For this review, take the finished solid that the model builds, in its own axes (mm). A direction names the side the tool comes from. Coordinates: 2 decimals unless noted, no trailing zeros. Loops run counter-clockwise (first coordinate to the right, second up) from the corner with the lowest first, then second, coordinate; pieces in that order, holes last. Notation, with made-up numbers: (26.25, -19) -> (74.25, -19) arc R11 ccw to (74.25, -3) -> close; hole circle Ø4 at (47, 80.25). An arc over 180 degrees is marked (long way). Use a Markdown table: item, result.
from build123d import *

# Parameters (mm, degrees)
BOSS_EXTRUDE1_DEPTH = 8


with BuildPart() as part:
    # Sketch1 → Boss-Extrude1 (new body)
    with BuildSketch(Plane(origin=(0, 0, 0), x_dir=(1, 0, 0), z_dir=(0, 1, 0))):
        with BuildLine():
            Line((-6, 6), (6, 6))
            ThreePointArc((6, 6), (12, 0), (6, -6))
            Line((6, -6), (-6, -6))
            ThreePointArc((-6, -6), (-12, 0), (-6, 6))
        make_face()
        Polygon((-4.63382, 3.298250285), (-7.36618, 3.298250285), (-9.298250285, 1.36618), (-9.298250285, -1.36618), (-7.36618, -3.298250285), (-4.63382, -3.298250285), (-2.701749715, -1.36618), (-2.701749715, 1.36618), align=None, mode=Mode.SUBTRACT)
        Polygon((8.355898234, 0.975845), (6.975845, 2.355898234), (5.024155, 2.355898234), (3.644101766, 0.975845), (3.644101766, -0.975845), (5.024155, -2.355898234), (6.975845, -2.355898234), (8.355898234, -0.975845), align=None, mode=Mode.SUBTRACT)
    extrude(amount=BOSS_EXTRUDE1_DEPTH)


solid = part.part
(1) For pin 1 Ø1.5 at (x, z) = (-6.5, -3.5) entering from -Y; pin 2 Ø4 at (x, y) = (9.5, 4.5) entering from +Z; pin 3 Ø1 at (x, z) = (-7, 2) entering from -Y; pin 4 Ø0.6 at (y, z) = (3.5, -0.5) entering from +X, all flat-tipped, find the tip position at first contact; note any pin that passes through.
Found:
| item | result |
|---|---|
| pin 1 | stops at y = 0 |
| pin 2 | stops at z = 5.81 |
| pin 3 | passes through |
| pin 4 | stops at x = 12 |
(2) Take a section at D-D on z = 2.75. Write out the cut boundary in (x, y).
Found:
| item | result |
|---|---|
| outline | (-11.33, 0) -> (-7.91, 0) -> (-7.91, 8) -> (-11.33, 8) -> close; (-4.09, 0) -> (11.33, 0) -> (11.33, 8) -> (-4.09, 8) -> close |
(3) For line 1 along X through (y, z) = (7, -0.25); line 2 along Z through (x, y) = (6.25, 5.75); line 3 along X through (y, z) = (7, 1.75), list the stretches that pass through material, from the lowest coordinate up.
Found:
| item | result |
|---|---|
| line 1 | x = -11.99 to -9.3, -2.7 to 3.64, 8.36 to 11.99 |
| line 2 | z = -5.99 to -2.36, 2.36 to 5.99 |
| line 3 | x = -11.74 to -8.91, -3.09 to 4.42, 7.58 to 11.74 |
(4) Take a section at A-A on z = 0. Write out the cut boundary in (x, y), plus the area to 3 significant figures.
Found:
| item | result |
|---|---|
| outline | (-12, 0) -> (-9.3, 0) -> (-9.3, 8) -> (-12, 8) -> close; (-2.7, 0) -> (3.64, 0) -> (3.64, 8) -> (-2.7, 8) -> close; (8.36, 0) -> (12, 0) -> (12, 8) -> (8.36, 8) -> close |
| area | 102 mm^2 |
(5) For faces 1 (the face through (3.644, 4, 0)), 2 (the face through (12, 4, 0)), list the 3-axis set-ups (+Z, -Z, +X, -X, +Y, -Y) from which the entire face can be reached by the end or side of a thin tool; tool diameter is ignored.
Found:
| item | result |
|---|---|
| face 1 | +Y, -Y |
| face 2 | +X, +Y, -Y |
(6) Take a section at C-C on x = -8.25. Write out the cut boundary in (y, z), plus the area to 3 significant figures.
Found:
| item | result |
|---|---|
| outline | (0, -5.56) -> (8, -5.56) -> (8, -2.41) -> (0, -2.41) -> close; (0, 2.41) -> (8, 2.41) -> (8, 5.56) -> (0, 5.56) -> close |
| area | 50.4 mm^2 |
(7) Take a section at B-B on y = 2. Write out the cut boundary in (x, z).
Found:
| item | result |
|---|---|
| outline | (-6, -6) -> (6, -6) arc R6 ccw to (6, 6) -> (-6, 6) arc R6 ccw to start; hole (-9.3, -1.37) -> (-7.37, -3.3) -> (-4.63, -3.3) -> (-2.7, -1.37) -> (-2.7, 1.37) -> (-4.63, 3.3) -> (-7.37, 3.3) -> (-9.3, 1.37) -> close; hole (3.64, -0.98) -> (5.02, -2.36) -> (6.98, -2.36) -> (8.36, -0.98) -> (8.36, 0.98) -> (6.98, 2.36) -> (5.02, 2.36) -> (3.64, 0.98) -> close |
(8) Mouldability with a two-part tool opening along Z and no side actions: class faces 3 (the face through (0, 4, 6)), 4 (the face through (-2.702, 4, 0)), 5 (the face through (6, 4, 2.356)), 6 (the face through (-12, 4, 0)) as pulls with the +Z half, pulls with the -Z half, needs draft (parallel to the pull), parting line crosses it, or undercut.
Found:
| item | result |
|---|---|
| face 3 | pulls with the +Z half |
| face 4 | undercut |
| face 5 | undercut |
| face 6 | parting line crosses it |
